from build123d import *

# Parameters (mm, degrees)
SKETCH1_W                    = 120
SKETCH1_H                    = 70
BOSS_EXTRUDE1_DEPTH          = 34
SHELL1_T                     = -1.6
CUT_EXTRUDE1_REACH           = 79.337
SKETCH2_W                    = 76
SKETCH2_H                    = 66.8
SKETCH3_W                    = 1.6
SKETCH3_H                    = 70
BOSS_EXTRUDE2_DEPTH          = 4.5
SKETCH4_R                    = 3
CUT_EXTRUDE2_DEPTH           = 0.8
CUT_EXTRUDE3_REACH           = 79.337
SKETCH5_R                    = 2
SKETCH7_W                    = 71.2
SKETCH7_H                    = 66.8
SKETCH7_W_2                  = 38.8
SKETCH7_H_2                  = 55.6
BOSS_EXTRUDE3_DEPTH          = 1.6
CUT_EXTRUDE4_DEPTH           = 1.6
CUT_EXTRUDE4_DRAFT           = -45
CUT_EXTRUDE4_PROFILE_2_DEPTH = 1.6
CUT_EXTRUDE4_PROFILE_2_DRAFT = -45
CUT_EXTRUDE4_PROFILE_3_DEPTH = 1.6
CUT_EXTRUDE4_PROFILE_3_DRAFT = -45
CUT_EXTRUDE4_PROFILE_4_DEPTH = 1.6
CUT_EXTRUDE4_PROFILE_4_DRAFT = -45
CUT_EXTRUDE4_PROFILE_5_DEPTH = 1.6
CUT_EXTRUDE4_PROFILE_5_DRAFT = -45
CUT_EXTRUDE4_PROFILE_6_DEPTH = 1.6
CUT_EXTRUDE4_PROFILE_6_DRAFT = -45
CUT_EXTRUDE5_START           = -1.6
SKETCH9_W                    = 24
SKETCH9_H                    = 12
CUT_EXTRUDE5_DEPTH           = 0.8


with BuildPart() as part:
    # Sketch1 → Boss-Extrude1 (new body)
    with BuildSketch(Plane(origin=(0, 0, 0), x_dir=(1, 0, 0), z_dir=(0, 1, 0))):
        Rectangle(SKETCH1_W, SKETCH1_H)
    extrude(amount=BOSS_EXTRUDE1_DEPTH)

    # Shell1
    shell1_openings = [part.faces().sort_by_distance(p)[0] for p in [
        (0, 0, 0),
    ]]
    offset(amount=SHELL1_T, openings=shell1_openings, kind=Kind.INTERSECTION)

    # Sketch2 → Cut-Extrude1 (cut, up to next)
    with BuildSketch(Plane(origin=(0, 34, 0), x_dir=(1, 0, 0), z_dir=(0, 1, 0)), mode=Mode.PRIVATE) as cut_extrude1_sk1:
        Rectangle(SKETCH2_W, SKETCH2_H)
    cut_extrude1_tool1 = extrude(cut_extrude1_sk1.sketch, amount=-CUT_EXTRUDE1_REACH, mode=Mode.PRIVATE) & part.part
    add(cut_extrude1_tool1.solids().sort_by_distance((0, 34, 0))[0], mode=Mode.SUBTRACT)

    # Sketch3 → Boss-Extrude2 (add)
    with BuildSketch(Plane(origin=(0, 34, 0), x_dir=(1, 0, 0), z_dir=(0, 1, 0))):
        with Locations((-38.8, 0)):
            Rectangle(SKETCH3_W, SKETCH3_H)
    boss_extrude2 = extrude(amount=-BOSS_EXTRUDE2_DEPTH)

    # Sketch4 → Cut-Extrude2 (cut)
    with BuildSketch(Plane(origin=(0, 34, 0), x_dir=(1, 0, 0), z_dir=(0, 1, 0))):
        with Locations(Location((-42.5, 0, 0), (0, 0, 270))):
            Circle(SKETCH4_R)
    cut_extrude2 = extrude(amount=-CUT_EXTRUDE2_DEPTH, mode=Mode.SUBTRACT)

    # Sketch5 → Cut-Extrude3 (cut, up to next)
    with BuildSketch(Plane(origin=(0, 34, 0), x_dir=(1, 0, 0), z_dir=(0, 1, 0)), mode=Mode.PRIVATE) as cut_extrude3_sk1:
        with Locations(Location((-42.5, 0, 0), (0, 0, 270))):
            Circle(SKETCH5_R)
    cut_extrude3_tool1 = extrude(cut_extrude3_sk1.sketch, amount=-CUT_EXTRUDE3_REACH, mode=Mode.PRIVATE) & part.part
    cut_extrude3 = cut_extrude3_tool1.solids().sort_by_distance((-42.5, 34, 0))[0]
    add(cut_extrude3, mode=Mode.SUBTRACT)

    # Mirror1: Boss-Extrude2, Cut-Extrude2, Cut-Extrude3 across plane
    add(boss_extrude2.mirror(Plane(origin=(0, 0, 0), x_dir=(0, 0, 1), z_dir=(1, 0, 0))))
    add(cut_extrude2.mirror(Plane(origin=(0, 0, 0), x_dir=(0, 0, 1), z_dir=(1, 0, 0))), mode=Mode.SUBTRACT)
    add(cut_extrude3.mirror(Plane(origin=(0, 0, 0), x_dir=(0, 0, 1), z_dir=(1, 0, 0))), mode=Mode.SUBTRACT)

    # Sketch7 → Boss-Extrude3 (add)
    with BuildSketch(Plane(origin=(0, 0, 0), x_dir=(1, 0, 0), z_dir=(0, 1, 0))):
        Rectangle(SKETCH7_W, SKETCH7_H)
        Rectangle(SKETCH7_W_2, SKETCH7_H_2, mode=Mode.SUBTRACT)
    extrude(amount=BOSS_EXTRUDE3_DEPTH)


with BuildPart() as cut_extrude4_tool:
    # Sketch8 → Cut-Extrude4 (with draft: the straight prism first)
    with BuildSketch(Plane(origin=(0, 1.6, 0), x_dir=(1, 0, 0), z_dir=(0, 1, 0))):
        with BuildLine():
            ThreePointArc((-31.5, 3), (-34.5, 0), (-31.5, -3))
            Line((-31.5, -3), (-23.5, -3))
            ThreePointArc((-23.5, -3), (-20.5, 0), (-23.5, 3))
            Line((-23.5, 3), (-31.5, 3))
        make_face()
    extrude(amount=-CUT_EXTRUDE4_DEPTH)
    # Cut-Extrude4: the draft: its side faces are tilted about the plane it starts from
    cut_extrude4_sides = [cut_extrude4_tool.faces().sort_by_distance(p)[0] for p in [
        (-20.5, 0.8, 0),
        (-27.5, 0.8, -3),
        (-34.5, 0.8, 0),
        (-27.5, 0.8, 3),
    ]]
    draft(cut_extrude4_sides, Plane(origin=(0, 1.6, 0), x_dir=(1, 0, 0), z_dir=(0, 1, 0)), CUT_EXTRUDE4_DRAFT)


with BuildPart() as part_1:
    add(part.part)

    # Cut-Extrude4: cut by cut_extrude4_tool
    add(cut_extrude4_tool.part, mode=Mode.SUBTRACT)


with BuildPart() as cut_extrude4_profile_2_tool:
    # Sketch8 → Cut-Extrude4 profile 2 (with draft: the straight prism first)
    with BuildSketch(Plane(origin=(0, 1.6, 0), x_dir=(1, 0, 0), z_dir=(0, 1, 0))):
        with BuildLine():
            ThreePointArc((24.5, -4), (27.5, -7), (30.5, -4))
            Line((30.5, -4), (30.5, 4))
            ThreePointArc((30.5, 4), (27.5, 7), (24.5, 4))
            Line((24.5, 4), (24.5, -4))
        make_face()
    extrude(amount=-CUT_EXTRUDE4_PROFILE_2_DEPTH)
    # Cut-Extrude4 profile 2: the draft: its side faces are tilted about the plane it starts from
    cut_extrude4_profile_2_sides = [cut_extrude4_profile_2_tool.faces().sort_by_distance(p)[0] for p in [
        (27.5, 0.8, -7),
        (24.5, 0.8, 0),
        (27.5, 0.8, 7),
        (30.5, 0.8, 0),
    ]]
    draft(cut_extrude4_profile_2_sides, Plane(origin=(0, 1.6, 0), x_dir=(1, 0, 0), z_dir=(0, 1, 0)), CUT_EXTRUDE4_PROFILE_2_DRAFT)


with BuildPart() as part_2:
    add(part_1.part)

    # Cut-Extrude4 profile 2: cut by cut_extrude4_profile_2_tool
    add(cut_extrude4_profile_2_tool.part, mode=Mode.SUBTRACT)


with BuildPart() as cut_extrude4_profile_3_tool:
    # Sketch8 → Cut-Extrude4 profile 3 (with draft: the straight prism first)
    with BuildSketch(Plane(origin=(0, 1.6, 0), x_dir=(1, 0, 0), z_dir=(0, 1, 0))):
        with BuildLine():
            ThreePointArc((23.5, 22), (20.5, 19), (23.5, 16))
            Line((23.5, 16), (31.5, 16))
            ThreePointArc((31.5, 16), (34.5, 19), (31.5, 22))
            Line((31.5, 22), (23.5, 22))
        make_face()
    extrude(amount=-CUT_EXTRUDE4_PROFILE_3_DEPTH)
    # Cut-Extrude4 profile 3: the draft: its side faces are tilted about the plane it starts from
    cut_extrude4_profile_3_sides = [cut_extrude4_profile_3_tool.faces().sort_by_distance(p)[0] for p in [
        (34.5, 0.8, -19),
        (27.5, 0.8, -22),
        (20.5, 0.8, -19),
        (27.5, 0.8, -16),
    ]]
    draft(cut_extrude4_profile_3_sides, Plane(origin=(0, 1.6, 0), x_dir=(1, 0, 0), z_dir=(0, 1, 0)), CUT_EXTRUDE4_PROFILE_3_DRAFT)


with BuildPart() as part_3:
    add(part_2.part)

    # Cut-Extrude4 profile 3: cut by cut_extrude4_profile_3_tool
    add(cut_extrude4_profile_3_tool.part, mode=Mode.SUBTRACT)


with BuildPart() as cut_extrude4_profile_4_tool:
    # Sketch8 → Cut-Extrude4 profile 4 (with draft: the straight prism first)
    with BuildSketch(Plane(origin=(0, 1.6, 0), x_dir=(1, 0, 0), z_dir=(0, 1, 0))):
        with BuildLine():
            ThreePointArc((23.5, -16), (20.5, -19), (23.5, -22))
            Line((23.5, -22), (31.5, -22))
            ThreePointArc((31.5, -22), (34.5, -19), (31.5, -16))
            Line((31.5, -16), (23.5, -16))
        make_face()
    extrude(amount=-CUT_EXTRUDE4_PROFILE_4_DEPTH)
    # Cut-Extrude4 profile 4: the draft: its side faces are tilted about the plane it starts from
    cut_extrude4_profile_4_sides = [cut_extrude4_profile_4_tool.faces().sort_by_distance(p)[0] for p in [
        (34.5, 0.8, 19),
        (27.5, 0.8, 16),
        (20.5, 0.8, 19),
        (27.5, 0.8, 22),
    ]]
    draft(cut_extrude4_profile_4_sides, Plane(origin=(0, 1.6, 0), x_dir=(1, 0, 0), z_dir=(0, 1, 0)), CUT_EXTRUDE4_PROFILE_4_DRAFT)


with BuildPart() as part_4:
    add(part_3.part)

    # Cut-Extrude4 profile 4: cut by cut_extrude4_profile_4_tool
    add(cut_extrude4_profile_4_tool.part, mode=Mode.SUBTRACT)


with BuildPart() as cut_extrude4_profile_5_tool:
    # Sketch8 → Cut-Extrude4 profile 5 (with draft: the straight prism first)
    with BuildSketch(Plane(origin=(0, 1.6, 0), x_dir=(1, 0, 0), z_dir=(0, 1, 0))):
        with BuildLine():
            ThreePointArc((-30.5, 15), (-27.5, 12), (-24.5, 15))
            Line((-24.5, 15), (-24.5, 23))
            ThreePointArc((-24.5, 23), (-27.5, 26), (-30.5, 23))
            Line((-30.5, 23), (-30.5, 15))
        make_face()
    extrude(amount=-CUT_EXTRUDE4_PROFILE_5_DEPTH)
    # Cut-Extrude4 profile 5: the draft: its side faces are tilted about the plane it starts from
    cut_extrude4_profile_5_sides = [cut_extrude4_profile_5_tool.faces().sort_by_distance(p)[0] for p in [
        (-24.5, 0.8, -19),
        (-27.5, 0.8, -26),
        (-30.5, 0.8, -19),
        (-27.5, 0.8, -12),
    ]]
    draft(cut_extrude4_profile_5_sides, Plane(origin=(0, 1.6, 0), x_dir=(1, 0, 0), z_dir=(0, 1, 0)), CUT_EXTRUDE4_PROFILE_5_DRAFT)


with BuildPart() as part_5:
    add(part_4.part)

    # Cut-Extrude4 profile 5: cut by cut_extrude4_profile_5_tool
    add(cut_extrude4_profile_5_tool.part, mode=Mode.SUBTRACT)


with BuildPart() as cut_extrude4_profile_6_tool:
    # Sketch8 → Cut-Extrude4 profile 6 (with draft: the straight prism first)
    with BuildSketch(Plane(origin=(0, 1.6, 0), x_dir=(1, 0, 0), z_dir=(0, 1, 0))):
        with BuildLine():
            ThreePointArc((-30.5, -23), (-27.5, -26), (-24.5, -23))
            Line((-24.5, -23), (-24.5, -15))
            ThreePointArc((-24.5, -15), (-27.5, -12), (-30.5, -15))
            Line((-30.5, -15), (-30.5, -23))
        make_face()
    extrude(amount=-CUT_EXTRUDE4_PROFILE_6_DEPTH)
    # Cut-Extrude4 profile 6: the draft: its side faces are tilted about the plane it starts from
    cut_extrude4_profile_6_sides = [cut_extrude4_profile_6_tool.faces().sort_by_distance(p)[0] for p in [
        (-27.5, 0.8, 26),
        (-24.5, 0.8, 19),
        (-27.5, 0.8, 12),
        (-30.5, 0.8, 19),
    ]]
    draft(cut_extrude4_profile_6_sides, Plane(origin=(0, 1.6, 0), x_dir=(1, 0, 0), z_dir=(0, 1, 0)), CUT_EXTRUDE4_PROFILE_6_DRAFT)


with BuildPart() as part_6:
    add(part_5.part)

    # Cut-Extrude4 profile 6: cut by cut_extrude4_profile_6_tool
    add(cut_extrude4_profile_6_tool.part, mode=Mode.SUBTRACT)

    # Sketch9 → Cut-Extrude5 (cut)
    with BuildSketch(Plane.ZY.offset(60).offset(CUT_EXTRUDE5_START)):
        with Locations((0, 6)):
            Rectangle(SKETCH9_W, SKETCH9_H)
    cut_extrude5 = extrude(amount=CUT_EXTRUDE5_DEPTH, mode=Mode.SUBTRACT)

    # Mirror2: Cut-Extrude5 across plane
    add(cut_extrude5.mirror(Plane(origin=(0, 0, 0), x_dir=(0, 0, 1), z_dir=(1, 0, 0))), mode=Mode.SUBTRACT)


solid = part_6.part
Geometry check sheet. Reference: the model listing, model coordinates, mm. A direction names the side the tool comes from. Coordinates: 2 decimals unless noted, no trailing zeros. Order: outer loops, then holes, each group sorted by start corner. A loop starts at its lowest first (then second) coordinate and runs counter-clockwise, first axis right, second up. Notation, with made-up numbers: (4, 85.5) -> (14, 85.5) arc R17 cw to (14, 95.5) -> close; hole circle Ø4 at (83.5, 51.25). An arc over 180 degrees is marked (long way). Use a Markdown table: item, result. Add a question column.
1. Cross-section at B-B (y = 17). Enter the section's corners in (x, z), and give its area (3 significant figures).
2. Material ranges on L1, parallel to X at y = 33.8, z = 0; L2, parallel to Z at x = 42.5, y = 32.7; L3, parallel to Z at x = -12, y = 18.5, recorded low to high.
3. Cross-section at C-C (x = 27.5). Enter the section's corners in (y, z).
4. Go/stop test with flat-tipped pins: pin 1 Ø10 at (x, z) = (-17, 13.5) entering from +Y; pin 2 Ø5 at (x, z) = (42.5, 0) entering from -Y; pin 3 Ø10 at (x, z) = (-28, -23) entering from -Y. Record where each tip stops, or that it passes through.
5. Mould release check, pull along X, two halves, no side actions. Record for faces 1 (the face through (-60, 17, 0)), 2 (the face through (60, 17, 0)), 3 (the face through (-58.4, 16, 0)): pulls with the +X half, pulls with the -X half, needs draft (parallel to the pull), parting line crosses it, or undercut.
6. Cross-section at A-A (x = 9.5). Enter the section's corners in (y, z), and give its area (3 significant figures).
7. Set-up check for faces 4 (the face through (39.97, 33.61, 1.61)), 5 (the face through (44.452, 32.806, -0.434)), 6 (the face through (-39.6, 31, 0)), 7 (the face through (-1, 17, 33.4)): record each of +Z, -Z, +X, -X, +Y, -Y from which the full face is reachable in a straight line by a thin tool's end or side.
8. Cross-section at D-D (z = -30). Enter the section's corners in (x, y), and give its area (3 significant figures).
Filled sheet:
| question | item | result |
|---|---|---|
| 1 | outline | (-60, -35) -> (60, -35) -> (60, 35) -> (-60, 35) -> close; hole (-58.4, -33.4) -> (58.4, -33.4) -> (58.4, 33.4) -> (-58.4, 33.4) -> close |
| 1 | area | 598 mm2 |
| 2 | L1 | -60 to -45.5, -39.5 to -38, 38 to 39.5, 45.5 to 60 |
| 2 | L2 | -35 to -2, 2 to 35 |
| 2 | L3 | -35 to -33.4, 33.4 to 35 |
| 3 | outline | (0, -35) -> (34, -35) -> (34, -33.4) -> (1.6, -33.4) -> (1.6, -22) -> (0, -20.4) -> close; (0, -17.6) -> (1.6, -16) -> (1.6, -7) -> (0, -5.4) -> close; (0, 5.4) -> (1.6, 7) -> (1.6, 16) -> (0, 17.6) -> close; (0, 20.4) -> (1.6, 22) -> (1.6, 33.4) -> (34, 33.4) -> (34, 35) -> (0, 35) -> close |
| 4 | pin 1 | y = 1.6 |
| 4 | pin 2 | y = 32.4 |
| 4 | pin 3 | y = 0 |
| 5 | face 1 | pulls with the -X half |
| 5 | face 2 | pulls with the +X half |
| 5 | face 3 | undercut |
| 6 | outline | (0, -35) -> (34, -35) -> (34, -33.4) -> (1.6, -33.4) -> (1.6, -27.8) -> (0, -27.8) -> close; (0, 27.8) -> (1.6, 27.8) -> (1.6, 33.4) -> (34, 33.4) -> (34, 35) -> (0, 35) -> close |
| 6 | area | 127 mm2 |
| 7 | face 4 | +Y |
| 7 | face 5 | +Y, -Y |
| 7 | face 6 | -Y |
| 7 | face 7 | none |
| 8 | outline | (-60, 0) -> (-58.4, 0) -> (-58.4, 32.4) -> (-39.6, 32.4) -> (-39.6, 29.5) -> (-38, 29.5) -> (-38, 34) -> (-60, 34) -> close; (-35.6, 0) -> (35.6, 0) -> (35.6, 1.6) -> (-35.6, 1.6) -> close; (38, 29.5) -> (39.6, 29.5) -> (39.6, 32.4) -> (58.4, 32.4) -> (58.4, 0) -> (60, 0) -> (60, 34) -> (38, 34) -> close |
| 8 | area | 297 mm2 |
